```python
from build123d import *
from build123d.topology import SkipClean

# Parameters (mm, degrees)
SKETCH4_R            = 6.4
SKETCH4_R_2          = 2
BOSS_EXTRUDE3_DEPTH  = 1
BOSS_EXTRUDE6_START  = -3
SKETCH5_R            = 2
BOSS_EXTRUDE6_DEPTH  = 3.0001
BOSS_EXTRUDE22_REACH = 27.788
SKETCH9_R            = 6.419042014
BOSS_EXTRUDE9_DEPTH  = 1
BOSS_EXTRUDE23_REACH = 27.788


with BuildPart() as part:
    # Sketch3 → Revolve1 (revolve)
    with BuildSketch(Plane(origin=(0, 0, 0), x_dir=(0, 0, -1), z_dir=(1, 0, 0))):
        Polygon((-9, -1.5), (-4, -1), (-4, 1), (-9, 1.5), (-9, 4), (-2.4, 4), (-2.4, 6), (0, 6), (0, -6), (-2.4, -6), (-2.4, -4), (-9, -4), align=None)
    revolve(axis=Axis((0, 6, 0), (0, -1, 0)))



with BuildPart() as body_2:
    # Sketch4 → Boss-Extrude3 (new body)
    with BuildSketch(Plane(origin=(0, 4, 0), x_dir=(1, 0, 0), z_dir=(0, 1, 0))):
        with Locations(Location((0, 0, 0), (0, 0, 270))):
            Circle(SKETCH4_R)
        with Locations(Location((0, 0, 0), (0, 0, 270))):
            Circle(SKETCH4_R_2, mode=Mode.SUBTRACT)
    extrude(amount=BOSS_EXTRUDE3_DEPTH)


with BuildPart() as part_1:
    add(part.part)

    add(body_2.part)  # Boss-Extrude6 merges body 2
    # Sketch5 → Boss-Extrude6 (add)
    with BuildSketch(Plane(origin=(-6, 0, 3.854187267), x_dir=(0, 0, -1), z_dir=(1, 0, 0)).offset(BOSS_EXTRUDE6_START)):
        with BuildLine():
            ThreePointArc((21.854187267, -4), (25.854187267, 0), (21.854187267, 4))
            Line((21.854187267, 4), (3.854187267, 4))
            Line((3.854187267, 4), (3.854187267, -4))
            Line((3.854187267, -4), (21.854187267, -4))
        make_face()
        with Locations((21.854187267, 0)):
            Circle(SKETCH5_R, mode=Mode.SUBTRACT)
    boss_extrude6 = extrude(amount=BOSS_EXTRUDE6_DEPTH)

    # Mirror1: Boss-Extrude6 across plane
    add(boss_extrude6.mirror(Plane(origin=(0, 0, 0), x_dir=(0, 0, 1), z_dir=(1, 0, 0))))

    # Boss-Extrude22: up to this cone (the profile starts inside it)
    with SkipClean():  # the faces are left unmerged after this step: merging them gives an invalid solid
        boss_extrude22_end = Plane(origin=(0, -4, 0), z_dir=(0, -1, 0)).offset(-3.399999) * Cone(1e-05, 656.88, 65.687999, align=(Align.CENTER, Align.CENTER, Align.MIN), mode=Mode.PRIVATE)
        # Sketch18 → Boss-Extrude22 (add, up to the surface)
        with BuildSketch(Plane.XZ.offset(4), mode=Mode.PRIVATE) as boss_extrude22_sk1:
            Polygon((-6, -9.001972309), (5.9999, -9.001972309), (5.9999, -5.707140078), (-6, -5.888545051), align=None)
        boss_extrude22_tool1 = extrude(boss_extrude22_sk1.sketch, amount=-BOSS_EXTRUDE22_REACH, mode=Mode.PRIVATE) & boss_extrude22_end
        add(boss_extrude22_tool1.solids().sort_by_distance((0.056566, -4, -7.39948))[0])

    # Sketch9 → Boss-Extrude9 (add)
    with SkipClean():  # the faces are left unmerged after this step: merging them gives an invalid solid
        with BuildSketch(Plane(origin=(0, -4, 0), x_dir=(-1, 0, 0), z_dir=(0, -1, 0))):
            with Locations(Location((0, 0, 0), (0, 0, 90))):
                Circle(SKETCH9_R)
        extrude(amount=BOSS_EXTRUDE9_DEPTH)

    # Sketch11 → Cut-Revolve3 (revolve, cut)
    with SkipClean():  # the faces are left unmerged after this step: merging them gives an invalid solid
        with BuildSketch(Plane(origin=(0, 0, 0), x_dir=(0, 0, -1), z_dir=(1, 0, 0)), mode=Mode.PRIVATE) as cut_revolve3_sk:
            with BuildLine():
                ThreePointArc((-9, -1.5), (-10.657481343, 0), (-9, 1.5))
                Line((-9, 1.5), (-4, 1))
                Line((-4, 1), (-4, -1))
                Line((-4, -1), (-9, -1.5))
            make_face()
        revolve(cut_revolve3_sk.sketch.rotate(Axis((0, 6, 0), (0, -1, 0)), 180), axis=Axis((0, 6, 0), (0, -1, 0)), mode=Mode.SUBTRACT)

    # Boss-Extrude23: up to this cone (the profile starts inside it)
    boss_extrude23_end = Plane(origin=(0, 4, 0), z_dir=(0, 1, 0)).offset(-3.399999) * Cone(1e-05, 656.88, 65.687999, align=(Align.CENTER, Align.CENTER, Align.MIN), mode=Mode.PRIVATE)
    # Sketch22 → Boss-Extrude23 (add, up to the surface)
    with BuildSketch(Plane(origin=(0, 4, 0), x_dir=(1, 0, 0), z_dir=(0, 1, 0)), mode=Mode.PRIVATE) as boss_extrude23_sk1:
        Polygon((5.9999, 9.001972309), (-6, 9.001972309), (-6, 5.888545051), (5.9999, 5.707140078), align=None)
    boss_extrude23_tool1 = extrude(boss_extrude23_sk1.sketch, amount=-BOSS_EXTRUDE23_REACH, mode=Mode.PRIVATE) & boss_extrude23_end
    add(boss_extrude23_tool1.solids().sort_by_distance((0.056566, 4, -7.39948))[0])


solid = part_1.part
```
The listing builds one solid part. Answer for the finished solid, in the listing's coordinates (mm). A direction names the side the tool comes from. Give positions to 0.01 mm unless a question says otherwise; leave off trailing zeros. Order: outer loops, then holes, each group sorted by start corner. A loop starts at its lowest first (then second) coordinate and runs counter-clockwise, first axis right, second up. Notation, with made-up numbers: (-2, 58) -> (21, 58) arc R19 ccw to (21, 69) -> close; hole circle Ø7 at (57, 78). An arc over 180 degrees is marked (long way). Write each question's results on one line, items separated by ' | '.
Q1. Each of these flat-tipped pins is pushed along its axis until it touches: P1, Ø1.2, axis at x = -1, y = 3, coming from the -Z side; P2, Ø9, axis at x = 4, z = -8, coming from the +Y side; P3, Ø2.5, axis at x = -2, z = -6.5, coming from the -Y side. Where does it stop, or does it pass through?
Checked values:
P1: stops at z = -9 | P2: stops at y = 5 | P3: stops at y = -5
Q2. Determine the mould class of faces 6 (the face through (9, 0, -11)), 7 (the face through (-7.5, -1.2, -16.4)), 8 (the face through (-2.024, -5.493, 1.29)), 9 (the face through (6, 0, -14)) for opening direction X: pulls with the +X half, pulls with the -X half, needs draft (parallel to the pull), parting line crosses it, or undercut.
Checked values:
face 6: pulls with the +X half | face 7: needs draft | face 8: parting line crosses it | face 9: undercut
Q3. The part is cut by section B-B, the plane y = 0. Give the vertices of the cut face in (x, z).
Checked values:
outline: (-9, -22) -> (-6, -22) -> (-6, -20) -> (-9, -20) -> close; (-9, -16) -> (-6, -16) -> (-6, -8.81) arc R10.66 cw to (-9, -5.71) -> close; circle Ø8 at (0, 0); (6, -22) -> (9, -22) -> (9, -20) -> (6, -20) -> close; (6, -16) -> (9, -16) -> (9, -5.71) arc R10.66 cw to (6, -8.81) -> close
Q4. The part is cut by section A-A, the plane z = -11. Give the vertices of the cut face in (x, y).
Checked values:
outline: (-9, -4) -> (-6, -4) -> (-6, 4) -> (-9, 4) -> close; (6, -4) -> (9, -4) -> (9, 4) -> (6, 4) -> close
Q5. Straight lines are drawn through the part: probe 1 along X at (y, z) = (-3.75, -17); probe 2 along Y at (x, z) = (7, -18); probe 3 along Y at (x, z) = (-0.5, 4). For each, find the intervals that lie inside material, in ascending order. Write a range as from..to.
Checked values:
probe 1: x = -9..-6, 6..9 | probe 2: y = -4..-2, 2..4 | probe 3: y = -5..-1, 1..5
Q6. Which of the six approach directions +Z, -Z, +X, -X, +Y, -Y give full straight-line access (tool end or side, diameter ignored) to faces 1 (the face through (-2.46, -4.49, -5.93)), 2 (the face through (8, 0, -22)), 3 (the face through (0, 6, 0)), 4 (the face through (0, 4, -8)), 5 (the face through (0, 3, -9.002))?
Checked values:
face 1: -Y | face 2: -Z, +X, -X | face 3: +Z, -Z, +X, -X, +Y | face 4: +Y | face 5: -Z, +Y, -Y
Q7. The part is cut by section C-C, the plane z = -19. Give the vertices of the cut face in (x, y).
Checked values:
outline: (-9, -3.87) -> (-6, -3.87) -> (-6, -1.73) -> (-9, -1.73) -> close; (-9, 1.73) -> (-6, 1.73) -> (-6, 3.87) -> (-9, 3.87) -> close; (6, -3.87) -> (9, -3.87) -> (9, -1.73) -> (6, -1.73) -> close; (6, 1.73) -> (9, 1.73) -> (9, 3.87) -> (6, 3.87) -> close
